Read the model definition and answer for the solid it produces. Units are mm, in the model's axes. A direction names the side the tool comes from. Give positions to 0.01 mm unless a question says otherwise; leave off trailing zeros. Write each loop counter-clockwise with the first axis right and the second up, starting at its lowest first coordinate (ties: lowest second). Pieces come first, ordered by that corner, then holes. Notation, with made-up numbers: (-26, -5) - (-19, -5) arc R27 ccw to (-19, 26) - close; hole circle Ø10 at (86.25, 76.25). An arc over 180 degrees is marked (long way). Answer as CSV lines item,"result".
```python
from build123d import *

# Parameters (mm, degrees)
ESQUISSE1_R        = 2.5
BOSS_EXTRU_1_DEPTH = 2.4
ESQUISSE4_W        = 50.056999207
ESQUISSE4_H        = 2.995999995
BOSS_EXTRU_2_DEPTH = 36
BOSS_EXTRU_3_START = -15
ESQUISSE5_W        = 4.7
ESQUISSE5_H        = 11.59
ESQUISSE5_R        = 1
ESQUISSE5_W_2      = 7
ESQUISSE5_H_2      = 11.59300438
BOSS_EXTRU_3_DEPTH = 3
ESQUISSE6_W        = 6.951967
ESQUISSE6_H        = 11.62400213
BOSS_EXTRU_4_DEPTH = 3


with BuildPart() as part:
    # Esquisse1 → Boss.-Extru.1 (new body)
    with BuildSketch(Plane.XY):
        with BuildLine():
            Line((-39.447248325, 12.128903773), (10.609750882, 12.128903773))
            Line((10.609750882, 12.128903773), (10.609750882, 9.132903778))
            Line((10.609750882, 9.132903778), (0.375600944, 9.132903778))
            Line((0.375600944, 9.132903778), (4.304312905, 2.649911034))
            ThreePointArc((4.304312905, 2.649911034), (3.248571469, -3.872456776), (-3.358011614, -3.777948659))
            Line((-3.358011614, -3.777948659), (-13.470694005, 9.132903778))
            Line((-13.470694005, 9.132903778), (-39.447248325, 9.132903778))
            Line((-39.447248325, 9.132903778), (-39.447248325, 12.128903773))
        make_face()
        Circle(ESQUISSE1_R, mode=Mode.SUBTRACT)
    extrude(amount=BOSS_EXTRU_1_DEPTH)

    # Esquisse4 → Boss.-Extru.2 (add)
    with BuildSketch(Plane.XY.offset(2.4)):
        with Locations((-14.418748722, 10.630903776)):
            Rectangle(ESQUISSE4_W, ESQUISSE4_H)
    extrude(amount=BOSS_EXTRU_2_DEPTH)

    # Esquisse5 → Boss.-Extru.3 (add)
    # profile 1 of 2: a face of its own
    with BuildSketch(Plane.XY.offset(38.4).offset(BOSS_EXTRU_3_START)):
        with Locations((8.259750882, 3.337903778)):
            Rectangle(ESQUISSE5_W, ESQUISSE5_H)
        with Locations((8.5, 0)):
            Circle(ESQUISSE5_R, mode=Mode.SUBTRACT)
    # profile 2 of 2: a face of its own
    with BuildSketch(Plane.XY.offset(38.4).offset(BOSS_EXTRU_3_START)):
        with Locations((-21.190248118, 3.336401588)):
            Rectangle(ESQUISSE5_W_2, ESQUISSE5_H_2)
        with Locations((-19.5, 0)):
            Circle(ESQUISSE5_R, mode=Mode.SUBTRACT)
    extrude(amount=-BOSS_EXTRU_3_DEPTH)

    # Esquisse6 → Boss.-Extru.4 (add)
    with BuildSketch(Plane(origin=(-39.447248325, 0, -39.447248325), x_dir=(0, 0, -1), z_dir=(1, 0, 0))):
        with Locations((-49.047247825, 3.320902713)):
            Rectangle(ESQUISSE6_W, ESQUISSE6_H)
        with Locations((-68.247248825, 3.320902713)):
            Rectangle(ESQUISSE6_W, ESQUISSE6_H)
    extrude(amount=BOSS_EXTRU_4_DEPTH)


solid = part.part
```
(1) A cutting plane is placed at A-A (x = 8.5). Write down the section's boundary in (y, z).
Worked out:
outline,"(-2.46, 20.4) - (-1, 20.4) - (-1, 23.4) - (-2.46, 23.4) - close; (1, 20.4) - (9.13, 20.4) - (9.13, 0) - (12.13, 0) - (12.13, 38.4) - (9.13, 38.4) - (9.13, 23.4) - (1, 23.4) - close"
(2) Find the intervals of material crossed by L1, parallel to X at y = 8.5, z = 22; L2, parallel to Y at x = 8.5, z = 21.1; L3, parallel to Y at x = -12, z = 32, in increasing order.
Worked out:
L1,"x = -24.69 to -17.69, 5.91 to 10.61"
L2,"y = -2.46 to -1, 1 to 12.13"
L3,"y = 9.13 to 12.13"
(3) A cutting plane is placed at C-C (y = 0). Count the separate pieces of the cut face and the enclosed holes in it, and give its area (3 significant figures).
Worked out:
separate pieces,"8"
enclosed holes,"0"
area,"80.1 mm^2"
(4) A cutting plane is placed at B-B (y = 5). Write down the section's boundary in (x, z), and give its area (3 significant figures).
Worked out:
outline,"(-39.45, 6.12) - (-36.45, 6.12) - (-36.45, 13.08) - (-39.45, 13.08) - close; (-39.45, 25.32) - (-36.45, 25.32) - (-36.45, 32.28) - (-39.45, 32.28) - close; (-24.69, 20.4) - (-17.69, 20.4) - (-17.69, 23.4) - (-24.69, 23.4) - close; (-10.23, 0) - (2.88, 0) - (2.88, 2.4) - (-10.23, 2.4) - close; (5.91, 20.4) - (10.61, 20.4) - (10.61, 23.4) - (5.91, 23.4) - close"
area,"108 mm^2"
(5) The mould has two halves that part along Y. Classify faces 1 (the flat face through (-8.344, 2.587, 1.183)), 2 (the cylindrical face through (-20.5, 0, 21.9)), 3 (the flat face through (-2, 4, 2.4)): +Y half, -Y half, draft (parallel to the pull), parting line (faces both ways), or undercut.
Worked out:
face 1,"-Y half"
face 2,"undercut"
face 3,"draft"
(6) A cutting plane is placed at D-D (z = 12.5). Write down the section's boundary in (x, y).
Worked out:
outline,"(-39.45, -2.49) - (-36.45, -2.49) - (-36.45, 9.13) - (10.61, 9.13) - (10.61, 12.13) - (-39.45, 12.13) - close"
(7) Each of these flat-tipped pins is pushed along its axis until it touches: P1, Ø2.5, axis at x = 8, z = 22, coming from the -Y side; P2, Ø2, axis at x = -7.5, y = 6.5, coming from the +Z side; P3, Ø0.9, axis at y = 1.5, z = 22, coming from the -X side. Where does it stop, or does it pass through?
Worked out:
P1,"stops at y = -2.46"
P2,"stops at z = 2.4"
P3,"stops at x = -24.69"
(8) For faces 4 (the flat face through (-24.69, 3, 22)), 5 (the flat face through (8, 3, 23.4)), 6 (the flat face through (2.31, 5.94, 1.18)), 7 (the flat face through (-38, 3, 13.076)), determine the directions among +Z, -Z, +X, -X, +Y, -Y from which every point of the face is accessible in a straight line to the end or side of a thin tool.
Worked out:
face 4,"+Z, -Z, -X, -Y"
face 5,"+Z, +X, -X, -Y"
face 6,"+Z, -Z, +X"
face 7,"+X, -X, -Y"
